from build123d import *

# Parameters (mm, degrees)
BOSS_EXTRU_1_DEPTH = 5
CONG_1_R           = 2


with BuildPart() as part:
    # Esquisse1 → Boss.-Extru.1 (new body)
    with BuildSketch(Plane.XY):
        Polygon((30.3, 15.7), (30.3, 0), (205.7, 0), (205.7, 15.7), (205.7, 30.7), (220.7, 30.7), (236, 30.7), (236, 65.2), (162, 65.2), (162, 105.2), (74, 105.2), (74, 65.2), (0, 65.2), (0, 30.7), (15.3, 30.7), (30.3, 30.7), align=None)
        with BuildLine():
            ThreePointArc((15.3, 30.7), (25.906601718, 26.306601718), (30.3, 15.7))
            Line((30.3, 15.7), (30.3, 30.7))
            Line((30.3, 30.7), (15.3, 30.7))
        make_face()
        with BuildLine():
            Line((205.7, 30.7), (205.7, 15.7))
            ThreePointArc((205.7, 15.7), (210.093398282, 26.306601718), (220.7, 30.7))
            Line((220.7, 30.7), (205.7, 30.7))
        make_face()
    extrude(amount=BOSS_EXTRU_1_DEPTH)

    # Congé1
    cong_1_edges = [part.edges().sort_by_distance(p)[0] for p in [
        (205.7, 0, 2.5),
        (30.3, 0, 2.5),
        (0, 30.7, 2.5),
        (0, 65.2, 2.5),
        (236, 65.2, 2.5),
        (236, 30.7, 2.5),
    ]]
    fillet(cong_1_edges, radius=CONG_1_R)


solid = part.part
For this review, take the finished solid that the model builds, in its own axes (mm). A direction names the side the tool comes from. Give positions to 0.01 mm unless a question says otherwise; leave off trailing zeros. Loops run counter-clockwise (first coordinate to the right, second up) from the corner with the lowest first, then second, coordinate; pieces in that order, holes last.
Item 1: Insertion check: pin 1 (2.5 mm diameter, centred on x = 41.5, z = 3.5, fed in from +Y); pin 2 (2.5 mm diameter, centred on x = 5.5, z = 3.5, fed in from -Y); pin 3 (1.5 mm diameter, centred on y = 11.5, z = 3, fed in from +X). Each pin has a flat end and moves straight along its axis. Give the tip position at first contact, or say it passes through.
Item 2: Take a section at A-A, the plane z = 2.25. State the section outline as (x, y) points, and give its area (3 significant figures).
Item 3: Take a section at C-C, the plane x = 184.5. State the section outline as (y, z) points.
Item 4: Take a section at B-B, the plane y = 6.5. State the section outline as (x, z) points.
Item 5: For line 1 along Y through (x, z) = (193, 1.35); line 2 along X through (y, z) = (70, 2.4); line 3 along Y through (x, z) = (11.5, 0.45), list the stretches that pass through material, from the lowest coordinate up.
Item 6: Tool access review of faces 1 (the flat face through (205.7, 9, 2)), 2 (the flat face through (74, 85, 2)), 3 (the flat face through (199, 65.2, 2)), 4 (the flat face through (9, 30.7, 2)): name each direction out of +Z, -Z, +X, -X, +Y, -Y from which nothing blocks a thin tool from reaching the whole face with its end or side.
Calculated:
1. pin 1: stops at y = 65.2
1. pin 2: stops at y = 30.7
1. pin 3: stops at x = 205.7
2. outline: (0, 32.7) arc R2 ccw to (2, 30.7) - (15.3, 30.7) arc R15 cw to (30.3, 15.7) - (30.3, 2) arc R2 ccw to (32.3, 0) - (203.7, 0) arc R2 ccw to (205.7, 2) - (205.7, 15.7) arc R15 cw to (220.7, 30.7) - (234, 30.7) arc R2 ccw to (236, 32.7) - (236, 63.2) arc R2 ccw to (234, 65.2) - (162, 65.2) - (162, 105.2) - (74, 105.2) - (74, 65.2) - (2, 65.2) arc R2 ccw to (0, 63.2) - close
2. area: 17,100 mm2
3. outline: (0, 0) - (65.2, 0) - (65.2, 5) - (0, 5) - close
4. outline: (30.3, 0) - (205.7, 0) - (205.7, 5) - (30.3, 5) - close
5. line 1: y = 0 to 65.2
5. line 2: x = 74 to 162
5. line 3: y = 30.7 to 65.2
6. face 1: +Z, -Z, +X, -Y
6. face 2: +Z, -Z, -X, +Y
6. face 3: +Z, -Z, +X, +Y
6. face 4: +Z, -Z, -X, -Y
